Geometry check sheet. Reference: the model listing, model coordinates, mm. Face numbers are marked on the shaded views. A direction names the side the tool comes from. Coordinates: 2 decimals unless noted, no trailing zeros. Write each loop counter-clockwise with the first axis right and the second up, starting at its lowest first coordinate (ties: lowest second). Pieces come first, ordered by that corner, then holes. Notation, with made-up numbers: (4.25, -18.5) -> (14.25, -18.5) arc R29 ccw to (14.25, 13.5) -> close; hole circle Ø7 at (29, -36). An arc over 180 degrees is marked (long way). Answer in a Markdown table with one row per item. Add a question column.
1. Cross-section at C-C on x = 0. Record the cut outline in (y, z).
2. Cross-section at A-A on z = -11.5. Record the cut outline in (x, y), and give its area (3 significant figures).
3. Set-up check for the marked faces 1, 2, 3 and 4: record each of +Z, -Z, +X, -X, +Y, -Y from which the full face is reachable in a straight line by a thin tool's end or side.
4. Cross-section at B-B on z = -7.25. Record the cut outline in (x, y).
5. Mould release check, pull along X, two halves, no side actions. Record for the marked faces 5, 6 and 7: pulls with the +X half, pulls with the -X half, needs draft (parallel to the pull), parting line crosses it, or undercut.
6. Depth check by flat-ended pin: P1, Ø9.5, axis at x = 15, y = 5, coming from the +Z side; P2, Ø1.8, axis at x = -14.5, y = -6, coming from the +Z side; P3, Ø5.5, axis at x = 2, y = 0.5, coming from the -Z side. Enter the tip coordinate at first touch or a pass-through.
7. Scan lines: L1, parallel to Y at x = 15, z = -2.5; L2, parallel to Y at x = 15, z = -11.45; L3, parallel to X at y = 0, z = -5. Record each from-to range of solid material in increasing order. Write a range as from..to.
8. Cross-section at D-D on x = 12.5. Record the cut outline in (y, z).
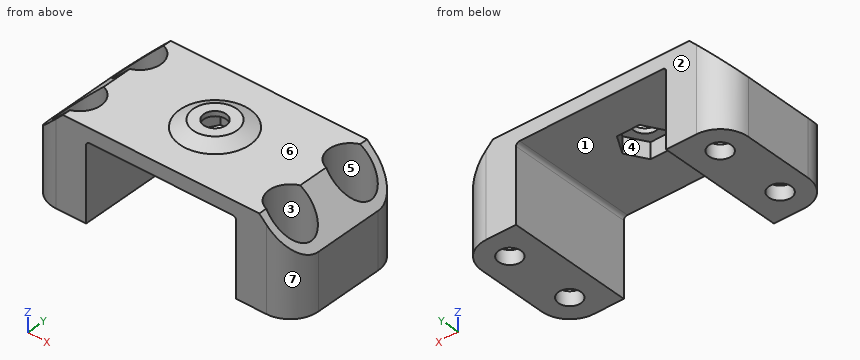
```python
from build123d import *

# Parameters (mm, degrees)
BOSS_EXTRUDE1_DEPTH     = 9
SKETCH2_R               = 1.6
CUT_EXTRUDE1_DEPTH      = 14
SKETCH3_R               = 1.6
CUT_EXTRUDE2_DEPTH      = 3
CUT_EXTRUDE3_DEPTH      = 2.3
CUT_EXTRUDE4_DEPTH      = 10
CUT_EXTRUDE4_DEPTH_BACK = 10
FILLET2_R               = 4
FILLET5_R               = 0.5
SKETCH11_R              = 3
CUT_EXTRUDE5_DEPTH      = 11


with BuildPart() as part:
    # Sketch1 → Boss-Extrude1 (new body, symmetric)
    with BuildSketch(Plane(origin=(0, 0, 0), x_dir=(1, 0, 0), z_dir=(0, 1, 0))):
        Polygon((10.7, 13), (19, 13), (19, 0), (-19, 0), (-19, 13), (-10.7, 13), (-10.7, 2), (10.7, 2), align=None)
    extrude(amount=BOSS_EXTRUDE1_DEPTH, both=True)

    # Sketch2 → Cut-Extrude1 (cut, through all)
    with BuildSketch(Plane(origin=(0, 0, -13), x_dir=(-1, 0, 0), z_dir=(0, 0, -1))):
        with Locations((-15, 5)):
            Circle(SKETCH2_R)
        with Locations((-15, -5)):
            Circle(SKETCH2_R)
        with Locations((15, 5)):
            Circle(SKETCH2_R)
        with Locations((15, -5)):
            Circle(SKETCH2_R)
    extrude(amount=-CUT_EXTRUDE1_DEPTH, mode=Mode.SUBTRACT)

    # Sketch3 → Cut-Extrude2 (cut, through all)
    with BuildSketch(Plane(origin=(0, 0, -2), x_dir=(-1, 0, 0), z_dir=(0, 0, -1))):
        Circle(SKETCH3_R)
    extrude(amount=-CUT_EXTRUDE2_DEPTH, mode=Mode.SUBTRACT)

    # Sketch9 → Revolve1 (revolve)
    with BuildSketch(Plane(origin=(0, 0, 0), x_dir=(0, 0, -1), z_dir=(1, 0, 0))):
        Polygon((0, 1.6), (0, 5), (-1, 3.1), (-1, 1.6), align=None)
    revolve(axis=Axis((0, 0, 0), (0, 0, 1)))

    # Sketch4 → Cut-Extrude3 (cut)
    with BuildSketch(Plane(origin=(0, 0, -2), x_dir=(-1, 0, 0), z_dir=(0, 0, -1))):
        Polygon((1.602042514, 2.808343483), (-1.631075541, 2.791581257), (-3.233118056, -0.016762226), (-1.602042514, -2.808343483), (1.631075541, -2.791581257), (3.233118056, 0.016762226), align=None)
    extrude(amount=-CUT_EXTRUDE3_DEPTH, mode=Mode.SUBTRACT)

    # Sketch10 → Cut-Extrude4 (cut, two sides)
    with BuildSketch(Plane(origin=(0, 0, 0), x_dir=(1, 0, 0), z_dir=(0, 1, 0))) as cut_extrude4_sk:
        Polygon((-19, 0), (-19, 5), (-14, 0), align=None)
        Polygon((14, 0), (19, 0), (19, 5), align=None)
    extrude(amount=CUT_EXTRUDE4_DEPTH, mode=Mode.SUBTRACT)
    extrude(cut_extrude4_sk.sketch, amount=-CUT_EXTRUDE4_DEPTH_BACK, mode=Mode.SUBTRACT)

    # Fillet2
    fillet2_edges = [part.edges().sort_by_distance(p)[0] for p in [
        (-19, -9, -9),
        (-19, 9, -9),
        (19, -9, -9),
        (19, 9, -9),
    ]]
    fillet(fillet2_edges, radius=FILLET2_R)

    # Fillet5
    fillet5_edges = [part.edges().sort_by_distance(p)[0] for p in [
        (-10.7, 0, -2),
        (10.7, 0, -2),
    ]]
    fillet(fillet5_edges, radius=FILLET5_R)

    # Sketch11 → Cut-Extrude5 (cut)
    with BuildSketch(Plane.XY):
        with Locations((-15, 5)):
            Circle(SKETCH11_R)
        with Locations((-15, -5)):
            Circle(SKETCH11_R)
        with Locations((15, 5)):
            Circle(SKETCH11_R)
        with Locations((15, -5)):
            Circle(SKETCH11_R)
    extrude(amount=-CUT_EXTRUDE5_DEPTH, mode=Mode.SUBTRACT)


solid = part.part
```
Results found:
| question | item | result |
|---|---|---|
| 1 | outline | (-9, -2) -> (-2.8, -2) -> (-2.8, 0.3) -> (-1.6, 0.3) -> (-1.6, 1) -> (-3.1, 1) -> (-5, 0) -> (-9, 0) -> close; (1.6, 0.3) -> (2.8, 0.3) -> (2.8, -2) -> (9, -2) -> (9, 0) -> (5, 0) -> (3.1, 1) -> (1.6, 1) -> close |
| 2 | outline | (-19, -5) arc R4 ccw to (-15, -9) -> (-10.7, -9) -> (-10.7, 9) -> (-15, 9) arc R4 ccw to (-19, 5) -> close; (10.7, -9) -> (15, -9) arc R4 ccw to (19, -5) -> (19, 5) arc R4 ccw to (15, 9) -> (10.7, 9) -> close; hole circle Ø3.2 at (-15, -5); hole circle Ø3.2 at (-15, 5); hole circle Ø3.2 at (15, -5); hole circle Ø3.2 at (15, 5) |
| 2 | area | 253 mm^2 |
| 3 | face 1 | -Z, +Y, -Y |
| 3 | face 2 | +Z, -Z, +X, -X, +Y |
| 3 | face 3 | +Z |
| 3 | face 4 | -Z |
| 4 | outline | (-19, -5) arc R4 ccw to (-15, -9) -> (-10.7, -9) -> (-10.7, 9) -> (-15, 9) arc R4 ccw to (-19, 5) -> close; (10.7, -9) -> (15, -9) arc R4 ccw to (19, -5) -> (19, 5) arc R4 ccw to (15, 9) -> (10.7, 9) -> close; hole circle Ø6 at (-15, -5); hole circle Ø6 at (-15, 5); hole circle Ø6 at (15, -5); hole circle Ø6 at (15, 5) |
| 5 | face 5 | undercut |
| 5 | face 6 | needs draft |
| 5 | face 7 | pulls with the +X half |
| 6 | P1 | stops at z = 0 |
| 6 | P2 | stops at z = -11 |
| 6 | P3 | stops at z = -2 |
| 7 | L1 | y = -9..-8, -2..2, 8..9 |
| 7 | L2 | y = -9..-6.6, -3.4..3.4, 6.6..9 |
| 7 | L3 | x = -19..-10.7, 10.7..19 |
| 8 | outline | (-9, -13) -> (9, -13) -> (9, 0) -> (6.66, 0) -> (6.66, -11) -> (3.34, -11) -> (3.34, 0) -> (-3.34, 0) -> (-3.34, -11) -> (-6.66, -11) -> (-6.66, 0) -> (-9, 0) -> close |
